Check sheet for the modelled part. Datum: model origin and axes. Units: mm. A direction names the side the tool comes from. Round coordinates to 2 decimals unless told otherwise and drop trailing zeros. Order: outer loops, then holes, each group sorted by start corner. A loop starts at its lowest first (then second) coordinate and runs counter-clockwise, first axis right, second up. Notation, with made-up numbers: (83, -30.5) -> (141, -30.5) arc R35 cw to (141, 3.5) -> close; hole circle Ø7 at (69, 38). An arc over 180 degrees is marked (long way). Answer in a Markdown table with one row per item. Add a question column.
1. Material ranges on L1, parallel to Y at x = 61.5, z = 1.25; L2, parallel to Y at x = 59, z = 2.75; L3, parallel to X at y = -74.5, z = 13.75, recorded low to high. Write a range as from..to.
2. Sectioned sample at D-D, the plane y = -66. Record the boundary of the cut face in (x, z).
3. Access from +Z, -Z, +X, -X, +Y, -Y to the whole of each face (thin tool, end or side, straight path). Record for faces 1 (the flat face through (52, -67.09, 1)), 2 (the flat face through (52, -76, 16)), 3 (the flat face through (52, -51, 0)), 4 (the flat face through (52.87, -25.9, 16.5)), 5 (the cylindrical face through (67.071, -78.155, 8.619)).
4. Sectioned sample at C-C, the plane y = -34.5. Record the boundary of the cut face in (x, z).
5. Depth check by flat-ended pin: P1, Ø0.6, axis at x = 56.5, y = -76.5, coming from the +Z side; P2, Ø3, axis at x = 51.5, y = -61, coming from the -Z side; P3, Ø1.5, axis at x = 57.5, y = -61, coming from the +Z side. Enter the tip coordinate at first touch or a pass-through.
6. Sectioned sample at A-A, the plane x = 43. Record the boundary of the cut face in (y, z), then the cut area to 3 significant figures.
7. Draft check along X on faces 6 (the flat face through (66, -52, 17)), 7 (the flat face through (52, -28.616, 9)), 8 (the cylindrical face through (37.27, -78.19, 8.62)). Enter one of: +X half, -X half, draft (parallel to the pull), parting line (faces both ways), or undercut.
8. Sectioned sample at B-B, the plane z = 13.5. Record the boundary of the cut face in (x, y), then the cut area to 3 significant figures.
```python
from build123d import *

# Parameters (mm, degrees)
SKETCH_3_W          = 30.974653289306993
SKETCH_3_H          = 53.86877740136471
EXTRUDE_1_DEPTH     = 17
SKETCH_5_W          = 27.381586342504548
SKETCH_5_H          = 50.55917117672057
CUT_EXTRUDE_1_DEPTH = 15
SKETCH_6_W          = 27.381586342504548
SKETCH_6_H          = 2
EXTRUDE_2_DEPTH     = 14
SKETCH_9_W          = 27.3909573875588
SKETCH_9_H          = 1.7284906083583529
CUT_EXTRUDE_3_DEPTH = 1
SKETCH_10_W         = 12.935202359823364
SKETCH_10_H         = 2.000000000000007
EXTRUDE_4_DEPTH     = 1
FILLET_1_R          = 2
SKETCH_11_W         = 27.381586342504548
SKETCH_11_H         = 4
CUT_EXTRUDE_4_DEPTH = 10


with BuildPart() as part:
    # 草图3 → 凸台-拉伸1 (new body)
    with BuildSketch(Plane.XY):
        with Locations((52.15403343225914, -51.822040042061936)):
            Rectangle(SKETCH_3_W, SKETCH_3_H)
    extrude(amount=EXTRUDE_1_DEPTH)

    # 草图5 → 切除-拉伸1 (cut)
    with BuildSketch(Plane.XY.offset(17)):
        with Locations((52.10467994598998, -51.89572753809822)):
            Rectangle(SKETCH_5_W, SKETCH_5_H)
    extrude(amount=-CUT_EXTRUDE_1_DEPTH, mode=Mode.SUBTRACT)

    # 草图6 → 凸台-拉伸2 (add)
    with BuildSketch(Plane.XY.offset(2.0000000000000018)):
        with Locations((52.10467994598998, -27.616141949737933)):
            Rectangle(SKETCH_6_W, SKETCH_6_H)
        with Locations((52.10467994598998, -76.1753131264585)):
            Rectangle(SKETCH_6_W, SKETCH_6_H)
    extrude(amount=EXTRUDE_2_DEPTH)

    # 草图9 → 切除-拉伸3 (cut)
    with BuildSketch(Plane.XY.offset(17)):
        with Locations((52.109365468517105, -25.75189664555876)):
            Rectangle(SKETCH_9_W, SKETCH_9_H)
    extrude(amount=-CUT_EXTRUDE_3_DEPTH, mode=Mode.SUBTRACT)

    # 草图10 → 凸台-拉伸4 (add)
    with BuildSketch(Plane.XY.offset(16)):
        with Locations((59.33724298238482, -25.887651341379584)):
            Rectangle(SKETCH_10_W, SKETCH_10_H)
    extrude(amount=EXTRUDE_4_DEPTH)

    # 圆角1
    fillet_1_edges = [part.edges().sort_by_distance(p)[0] for p in [
        (67.64136007691263, -78.75642874274429, 8.5),
        (36.66670678760564, -78.75642874274429, 8.5),
        (36.66670678760564, -24.88765134137958, 8.5),
        (67.64136007691263, -24.88765134137958, 8.5),
    ]]
    fillet(fillet_1_edges, radius=FILLET_1_R)

    # 草图11 → 切除-拉伸4 (cut)
    with BuildSketch(Plane.XY.offset(2.0000000000000018)):
        with Locations((52.10467994598998, -34.82711454905556)):
            Rectangle(SKETCH_11_W, SKETCH_11_H)
        with Locations((52.10467994598998, -69.09032852544172)):
            Rectangle(SKETCH_11_W, SKETCH_11_H)
    extrude(amount=-CUT_EXTRUDE_4_DEPTH, mode=Mode.SUBTRACT)


solid = part.part
```
Answer key:
| question | item | result |
|---|---|---|
| 1 | L1 | y = -78.76..-71.09, -67.09..-36.83, -32.83..-24.89 |
| 1 | L2 | y = -78.76..-75.18, -28.62..-24.89 |
| 1 | L3 | x = 36.67..38.41, 65.8..67.64 |
| 2 | outline | (36.67, 0) -> (67.64, 0) -> (67.64, 17) -> (65.8, 17) -> (65.8, 2) -> (38.41, 2) -> (38.41, 17) -> (36.67, 17) -> close |
| 3 | face 1 | +Z, -Z |
| 3 | face 2 | +Z |
| 3 | face 3 | -Z, +X, -X, +Y, -Y |
| 3 | face 4 | +Z, +Y |
| 3 | face 5 | +Z, -Z, +X, -Y |
| 4 | outline | (36.67, 0) -> (38.41, 0) -> (38.41, 17) -> (36.67, 17) -> close; (65.8, 0) -> (67.64, 0) -> (67.64, 17) -> (65.8, 17) -> close |
| 5 | P1 | stops at z = 16 |
| 5 | P2 | stops at z = 0 |
| 5 | P3 | stops at z = 2 |
| 6 | outline | (-78.76, 0) -> (-71.09, 0) -> (-71.09, 2) -> (-75.18, 2) -> (-75.18, 16) -> (-77.18, 16) -> (-77.18, 17) -> (-78.76, 17) -> close; (-67.09, 0) -> (-36.83, 0) -> (-36.83, 2) -> (-67.09, 2) -> close; (-32.83, 0) -> (-24.89, 0) -> (-24.89, 16) -> (-28.62, 16) -> (-28.62, 2) -> (-32.83, 2) -> close |
| 6 | area | 196 mm² |
| 7 | face 6 | draft |
| 7 | face 7 | undercut |
| 7 | face 8 | -X half |
| 8 | outline | (36.67, -76.76) arc R2 ccw to (38.67, -78.76) -> (65.64, -78.76) arc R2 ccw to (67.64, -76.76) -> (67.64, -26.89) arc R2 ccw to (65.64, -24.89) -> (38.67, -24.89) arc R2 ccw to (36.67, -26.89) -> close; hole (38.41, -75.18) -> (65.8, -75.18) -> (65.8, -28.62) -> (38.41, -28.62) -> close |
| 8 | area | 390 mm² |
